Can you work these out from the model? Positions are in its coordinate system, mm. A direction names the side the tool comes from. Give positions to 0.01 mm unless a question says otherwise; leave off trailing zeros. Write each loop counter-clockwise with the first axis right and the second up, starting at its lowest first coordinate (ties: lowest second). Pieces come first, ordered by that corner, then holes. Notation, with made-up numbers: (-0.5, 52) -> (9.5, 52) arc R12 cw to (9.5, 73) -> close; hole circle Ø1 at (22.25, 31). An arc over 180 degrees is marked (long way). One line per item, written item: value.
from build123d import *

# Parameters (mm, degrees)
SKETCH1_R                 = 25
BOSS_EXTRUDE1_DEPTH       = 2.5
FILLET1_R                 = 1
BOSS_EXTRUDE9_DEPTH       = 15
BOSS_EXTRUDE11_DEPTH      = 6.3
BOSS_EXTRUDE11_DEPTH_BACK = 6.3
SKETCH5_R                 = 17
CUT_EXTRUDE3_DEPTH        = 6.3
CUT_EXTRUDE3_DEPTH_BACK   = 6.3
SKETCH6_R                 = 12


with BuildPart() as part:
    # Sketch1 → Boss-Extrude1 (new body)
    with BuildSketch(Plane(origin=(0, 0, 0), x_dir=(1, 0, 0), z_dir=(0, 1, 0))):
        with Locations(Location((0, 0, 0), (0, 0, 270))):
            Circle(SKETCH1_R)
    extrude(amount=BOSS_EXTRUDE1_DEPTH)

    # Boss-Extrude3 cone 1 section (through the dimple's axis) → Boss-Extrude3 (revolve)
    with BuildSketch(Plane(origin=(0, 2.5, 0), x_dir=(0, 0, -1), z_dir=(1, 0, 0))):
        Polygon((0, 0), (25, 0), (0, 4.408174518), align=None)
    revolve(axis=Axis((0, 2.5, 0), (0, 1, 0)))

    # Fillet1
    fillet1_edges = [part.edges().sort_by_distance(p)[0] for p in [
        (-25, 2.5, 0),
    ]]
    fillet(fillet1_edges, radius=FILLET1_R)

    # Sketch4 → Boss-Extrude9 (add)
    with BuildSketch(Plane(origin=(0, 4, 0), x_dir=(-1, 0, 0), z_dir=(0, 1, 0))):
        Polygon((-6.085829464, 6.143185176), (0, 16.013255457), (6.085829464, 6.143185176), (6.085829464, -6.143185176), (0, -16.013255457), (-6.085829464, -6.143185176), align=None)
    extrude(amount=BOSS_EXTRUDE9_DEPTH)

    # Sketch5 → Boss-Extrude11 (add, two sides: drawn at the far end of the back side and taken through both)
    with BuildSketch(Plane(origin=(0, 0, 0), x_dir=(0, 0, -1), z_dir=(1, 0, 0)).offset(-BOSS_EXTRUDE11_DEPTH_BACK)):
        with Locations((0, 24)):
            Circle(SKETCH5_R)
    extrude(amount=BOSS_EXTRUDE11_DEPTH + BOSS_EXTRUDE11_DEPTH_BACK)

    # Sketch6 → Cut-Extrude3 (cut, two sides: drawn at the far end of the back side and taken through both)
    with BuildSketch(Plane(origin=(0, 0, 0), x_dir=(0, 0, -1), z_dir=(1, 0, 0)).offset(-CUT_EXTRUDE3_DEPTH_BACK)):
        with Locations((0, 24)):
            Circle(SKETCH6_R)
    extrude(amount=CUT_EXTRUDE3_DEPTH + CUT_EXTRUDE3_DEPTH_BACK, mode=Mode.SUBTRACT)


solid = part.part
1) If we section it at C-C (y = 10.5): Write out the boundary of the cut face in (x, z), and give its area (3 significant figures).
Answer list:
outline: (-6.3, -10.33) -> (-3.5, -10.33) -> (0, -16.01) -> (3.5, -10.33) -> (6.3, -10.33) -> (6.3, 10.33) -> (3.5, 10.33) -> (0, 16.01) -> (-3.5, 10.33) -> (-6.3, 10.33) -> close
area: 300 mm^2
2) If we section it at B-B (y = 16): Write out the boundary of the cut face in (x, z).
Answer list:
outline: (-6.3, -15) -> (-0.62, -15) -> (0, -16.01) -> (0.62, -15) -> (6.3, -15) -> (6.3, -8.94) -> (-6.3, -8.94) -> close; (-6.3, 8.94) -> (6.3, 8.94) -> (6.3, 15) -> (0.62, 15) -> (0, 16.01) -> (-0.62, 15) -> (-6.3, 15) -> close
3) We'd pull the mould along Y, two halves only. Please class faces 1 (the face through (-6.3, 20, 12)), 2 (the face through (-6.086, 6, 0)), 3 (the face through (0, 0, 0)): released by +Y, released by -Y, zero draft, split by the parting line, or undercut.
Answer list:
face 1: zero draft
face 2: undercut
face 3: released by -Y
4) Will these pins go through, and if not, where does the flat tip stop? pin 1 (1.5 mm diameter, centred on x = 4, z = 3.5, fed in from +Y); pin 2 (17 mm diameter, centred on y = 28.5, z = 2.5, fed in from +X); pin 3 (3 mm diameter, centred on y = 15, z = -10, fed in from -X).
Answer list:
pin 1: stops at y = 40.78
pin 2: stops at x = 6.3
pin 3: stops at x = -6.3
5) For faces 4 (the face through (2.324, 9.51, -12.244)), 5 (the face through (6.8, 5.68, 1.51)), 6 (the face through (6.3, 20, 12)), which set-ups out of +Z, -Z, +X, -X, +Y, -Y let a thin tool reach every point of the face, with its end or its side?
Answer list:
face 4: -Z, +X
face 5: none
face 6: +Z, -Z, +X, +Y
6) If we section it at A-A (y = 24): Write out the boundary of the cut face in (x, z).
Answer list:
outline: (-6.3, -17) -> (6.3, -17) -> (6.3, -12) -> (-6.3, -12) -> close; (-6.3, 12) -> (6.3, 12) -> (6.3, 17) -> (-6.3, 17) -> close
7) I need wall thicknesses on L1, parallel to Y at x = -3, z = 0; L2, parallel to Y at x = 16, z = 0; L3, parallel to X at y = 13, z = -12. Which ranges of each line are inside material? Lowest first, please.
Answer list:
L1: y = 0 to 12, 36 to 41
L2: y = 0 to 4.09
L3: x = -6.3 to 6.3
